Answer from the drawing. Dimensions are ordinates in mm from the lowest x, y and z of the part. A direction names the side the tool comes from. Coordinates: 2 decimals unless noted, no trailing zeros. Order: outer loops, then holes, each group sorted by start corner. A loop starts at its lowest first (then second) coordinate and runs counter-clockwise, first axis right, second up. Notation, with made-up numbers: (35.5, 89) -> (71.5, 89) arc R22 cw to (71.5, 115) -> close; hole circle Ø9 at (80, -12). An arc over 180 degrees is marked (long way). Answer as a JSON object with one key per item and string values. Group by question number.
1) Section C-C on z = 2.5 is taken. Determine the outline of the cut face in (x, y).
2) Consider L1, parallel to X at y = 4.95, z = 14.6; L2, parallel to X at y = 4.95, z = 14; L3, parallel to Z at x = 9.5, y = 5.5. Determine where each line is inside the solid, lowest interval first.
3) Determine the mould class of the marked faces 1, 2, 3 and 4 for opening direction X: released by +X, released by -X, zero draft, split by the parting line, or undercut.
4) Given pin 1 (1 mm diameter, centred on y = 8.5, z = 8, fed in from +X); pin 2 (1.5 mm diameter, centred on y = 1, z = 10.5, fed in from +X), each flat-ended and moving along its own axis, determine where each tip first touches the part or whether it passes through.
5) A tool of negligible diameter and unlimited length cuts with its end or side. For the marked faces 5 and 6, from which of +Z, -Z, +X, -X, +Y, -Y can it reach the whole face along a straight path? Write none if from no direction.
6) Section A-A on x = 4.95 is taken. Determine the outline of the cut face in (y, z), and give its area (3 significant figures).
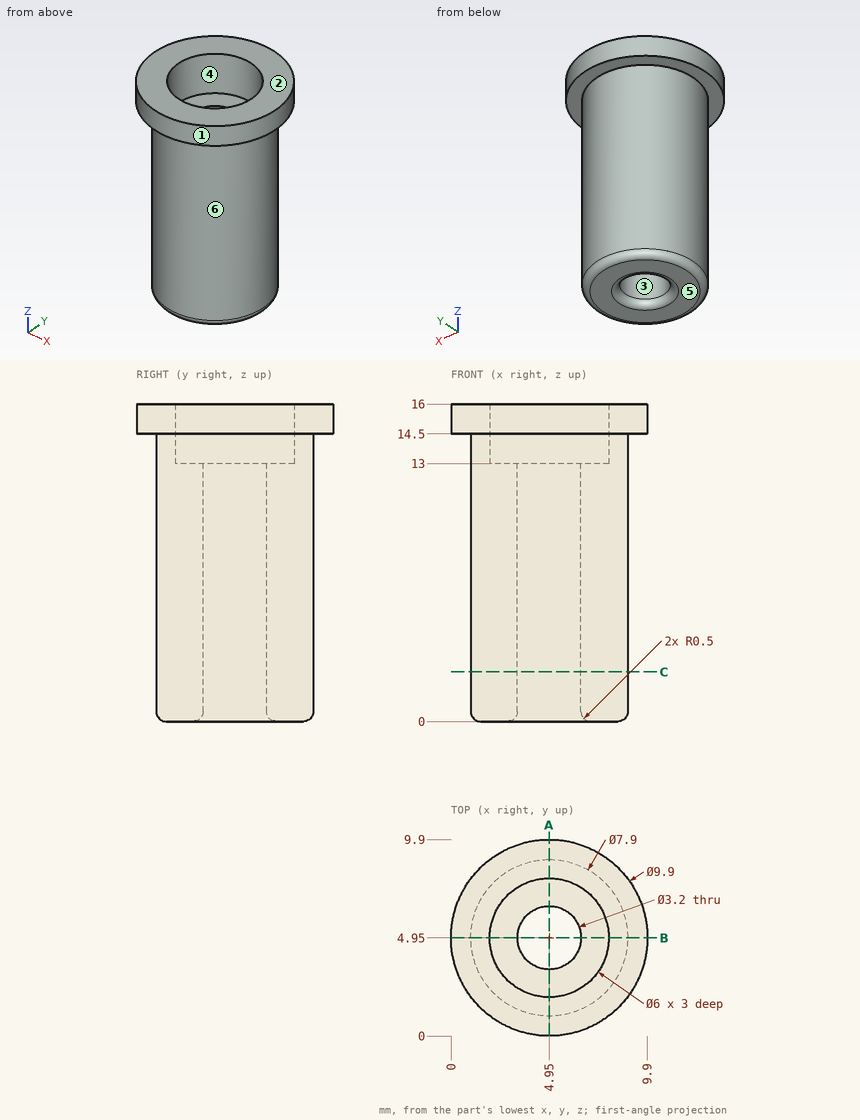
Worked answers:
{
 "1": {"outline": "circle Ø7.9 at (4.95, 4.95); hole circle Ø3.2 at (4.95, 4.95)"},
 "2": {"L1": "x = 0 to 1.95, 7.95 to 9.9", "L2": "x = 1 to 1.95, 7.95 to 8.9", "L3": "z = 14.5 to 16"},
 "3": {"face 1": "split by the parting line", "face 2": "zero draft", "face 3": "undercut", "face 4": "undercut"},
 "4": {"pin 1": "stops at x = 7.46", "pin 2": "stops at x = 7.27"},
 "5": {"face 5": "-Z, +X, -X, +Y, -Y", "face 6": "-Z"},
 "6": {"outline": "(0, 14.5) -> (1, 14.5) -> (1, 0.5) arc R0.5 ccw to (1.5, 0) -> (2.85, 0) arc R0.5 ccw to (3.35, 0.5) -> (3.35, 13) -> (1.95, 13) -> (1.95, 16) -> (0, 16) -> close; (6.55, 0.5) arc R0.5 ccw to (7.05, 0) -> (8.4, 0) arc R0.5 ccw to (8.9, 0.5) -> (8.9, 14.5) -> (9.9, 14.5) -> (9.9, 16) -> (7.95, 16) -> (7.95, 13) -> (6.55, 13) -> close", "area": "69.6 mm²"}
}
